Drawing for the job (mm, zero at the part's lowest x, y, z). A direction names the side the tool comes from. Give positions to 0.01 mm unless a question says otherwise; leave off trailing zeros. Loops run counter-clockwise (first coordinate to the right, second up) from the corner with the lowest first, then second, coordinate; pieces in that order, holes last. Notation, with made-up numbers: (73.25, -13.75) - (78.25, -13.75) arc R14 cw to (78.25, 12.25) - close; hole circle Ø10 at (23, 27). An arc over 180 degrees is marked (long way). Return JSON: item names as keys, results as strings. Group by question number.
1) Slice it at D-D (x = 2.75). List the corners of the cut face in (y, z).
2) Slice it at A-A (x = 11). List the corners of the cut face in (y, z).
3) Drop flat-ended pins along their axis: pin 1 (4 mm diameter, centred on x = 13.5, z = 14, fed in from +Y); pin 2 (10 mm diameter, centred on x = 10.5, z = 17.5, fed in from +Y). Give the stop position or say it passes through.
4) 3-axis set-ups, long thin cutter, end or side, ignore diameter. For the marked faces 1 and 2: which of +Z, -Z, +X, -X, +Y, -Y reach the whole face in a straight line?
5) Slice it at B-B (y = 10.25). List the corners of the cut face in (x, z).
6) Drill centre lines: probe 1 along Y at (x, z) = (7.5, 3); probe 2 along Z at (x, y) = (15.25, 8); probe 3 along Z at (x, y) = (11.25, 0.75). Where is each one in solid material? Low to high. Write a range as from..to.
7) Slice it at C-C (z = 13). List the corners of the cut face in (x, y).
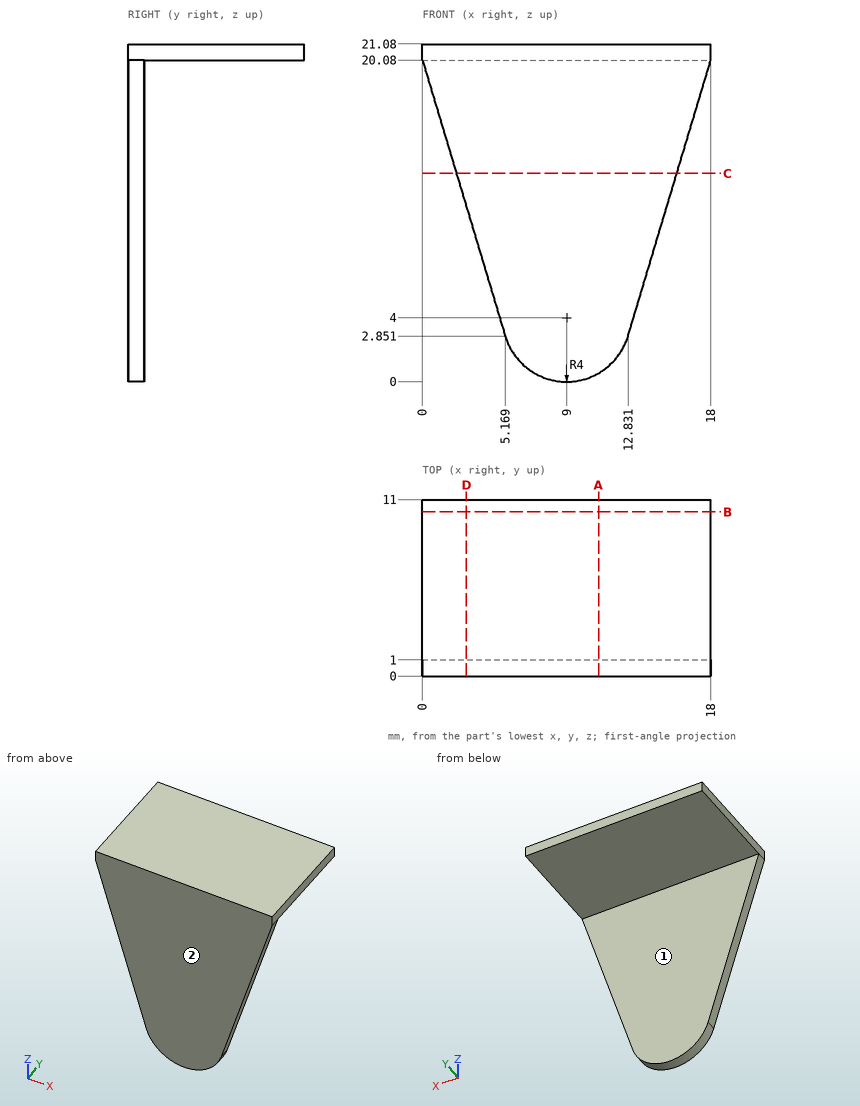
Results:
{
 "1": {"outline": "(0, 10.91) - (1, 10.91) - (1, 20.08) - (11, 20.08) - (11, 21.08) - (0, 21.08) - close"},
 "2": {"outline": "(0, 0.54) - (1, 0.54) - (1, 20.08) - (11, 20.08) - (11, 21.08) - (0, 21.08) - close"},
 "3": {"pin 1": "y = 1", "pin 2": "y = 11"},
 "4": {"face 1": "-Z, +X, -X, +Y", "face 2": "+Z, -Z, +X, -X, -Y"},
 "5": {"outline": "(0, 20.08) - (18, 20.08) - (18, 21.08) - (0, 21.08) - close"},
 "6": {"probe 1": "0..1", "probe 2": "20.08..21.08", "probe 3": "0.69..21.08"},
 "7": {"outline": "(2.12, 0) - (15.88, 0) - (15.88, 1) - (2.12, 1) - close"}
}
